Build history of the part. All positions in model axes, mm. Give positions to 0.01 mm unless a question says otherwise; leave off trailing zeros. Write each loop counter-clockwise with the first axis right and the second up, starting at its lowest first coordinate (ties: lowest second). Pieces come first, ordered by that corner, then holes. Notation, with made-up numbers: M 22.5,45.25 L 32.5,45.25 A28 ccw 32.5,75.25 Z; hole C 8.5,20 d11. An arc over 180 degrees is marked long. Return JSON: item names as keys, results as strings. Group by question number.
Q1. Wall check: probe 1 along X at (y, z) = (113, -1.8); probe 2 along X at (y, z) = (220, -2.25). Give the ranges that are in metal, low to high.
Q2. Flat gauge pins, fed straight in: pin 1 Ø1 at (y, z) = (115.5, -1) entering from +X; pin 2 Ø1.5 at (y, z) = (92, -2) entering from +X; pin 3 Ø1 at (y, z) = (195.5, -1) entering from +X. Where does each tip first touch, or does it go through?
Q3. Band-saw the part on A-A, the plane z = -0.55. Give the cut face in (x, y) (3 decimals), then the cut area to 3 significant figures.
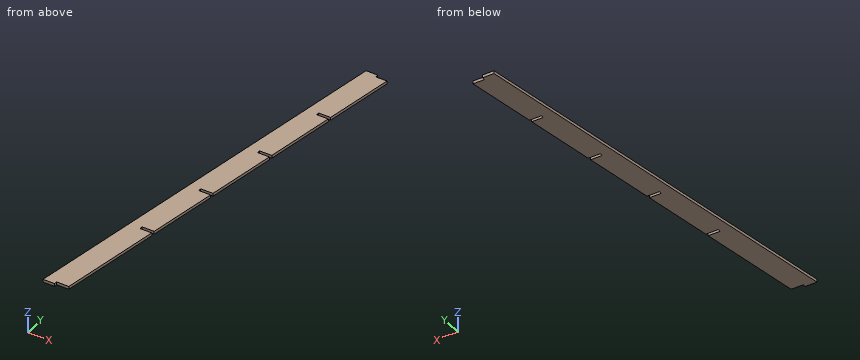
from build123d import *

# Parameters (mm, degrees)
SKETCH1_W          = 25.4
SKETCH1_H          = 3.175
SKETCH2_W          = 25.4
SKETCH2_H          = 3.175
CUT_EXTRUDE1_DEPTH = 5.08


with BuildPart() as part:
    # Sketch1 → Loft1 section 0
    with BuildSketch(Plane(origin=(0, 0, 0), x_dir=(1, 0, 0), z_dir=(0, 1, 0))):
        with Locations((12.7, 1.5875)):
            Rectangle(SKETCH1_W, SKETCH1_H)
    # Sketch2 → Loft1 section 1
    with BuildSketch(Plane(origin=(0, 432.562, 0), x_dir=(1, 0, 0), z_dir=(0, 1, 0))):
        with Locations((90.17, 1.5875)):
            Rectangle(SKETCH2_W, SKETCH2_H)
    loft()

    # Sketch3 → Cut-Extrude1 (cut)
    with BuildSketch(Plane.XY):
        Polygon((90.028717652, 432.562), (90.028717652, 429.26), (102.278625954, 429.26), (102.87, 432.562), align=None)
        Polygon((12.572909357, 3.175), (12.572909357, 0), (25.4, 0), (25.96862889, 3.175), align=None)
        Polygon((33.071424259, 117.475), (33.071424259, 114.3), (45.870640047, 114.3), (46.439268937, 117.475), align=None)
        Polygon((75.759721917, 353.738084411), (75.759721917, 350.595188566), (88.190095427, 350.595188566), (88.752974601, 353.738084411), align=None)
        Polygon((61.470871422, 274.955), (61.470871422, 271.78), (74.074633001, 271.78), (74.643261891, 274.955), align=None)
        Polygon((47.260398049, 193.04), (47.260398049, 196.215), (60.541265414, 196.215), (59.972636524, 193.04), align=None)
    extrude(amount=-CUT_EXTRUDE1_DEPTH, mode=Mode.SUBTRACT)


solid = part.part
From the geometry:
{
 "1": {"probe 1": "x = 20.24 to 45.64", "probe 2": "x = 39.4 to 64.8"},
 "2": {"pin 1": "stops at x = 33.07", "pin 2": "stops at x = 42.01", "pin 3": "stops at x = 47.26"},
 "3": {"outline": "M 0,0 L 12.573,0 L 12.573,3.175 L 25.969,3.175 L 45.871,114.3 L 33.071,114.3 L 33.071,117.475 L 46.439,117.475 L 59.973,193.04 L 47.26,193.04 L 47.26,196.215 L 60.541,196.215 L 74.075,271.78 L 61.471,271.78 L 61.471,274.955 L 74.643,274.955 L 88.19,350.595 L 75.76,350.595 L 75.76,353.738 L 88.753,353.738 L 102.279,429.26 L 90.029,429.26 L 90.029,432.562 L 77.47,432.562 Z", "area": "10,700 mm^2"}
}
